Geometry check sheet. Reference: drawing and pictorial views, mm from the part's lowest x, y, z. A direction names the side the tool comes from. Give positions to 0.01 mm unless a question says otherwise; leave off trailing zeros. Write each loop counter-clockwise with the first axis right and the second up, starting at its lowest first coordinate (ties: lowest second). Pieces come first, ordered by that corner, then holes. Notation, with made-up numbers: M 43.5,-2.75 L 101.5,-2.75 A17 ccw 101.5,16.25 Z; hole C 52,-31.75 d7. An arc over 180 degrees is marked long. Write each question's results on one line, items separated by ' | '. Start each with the question number.
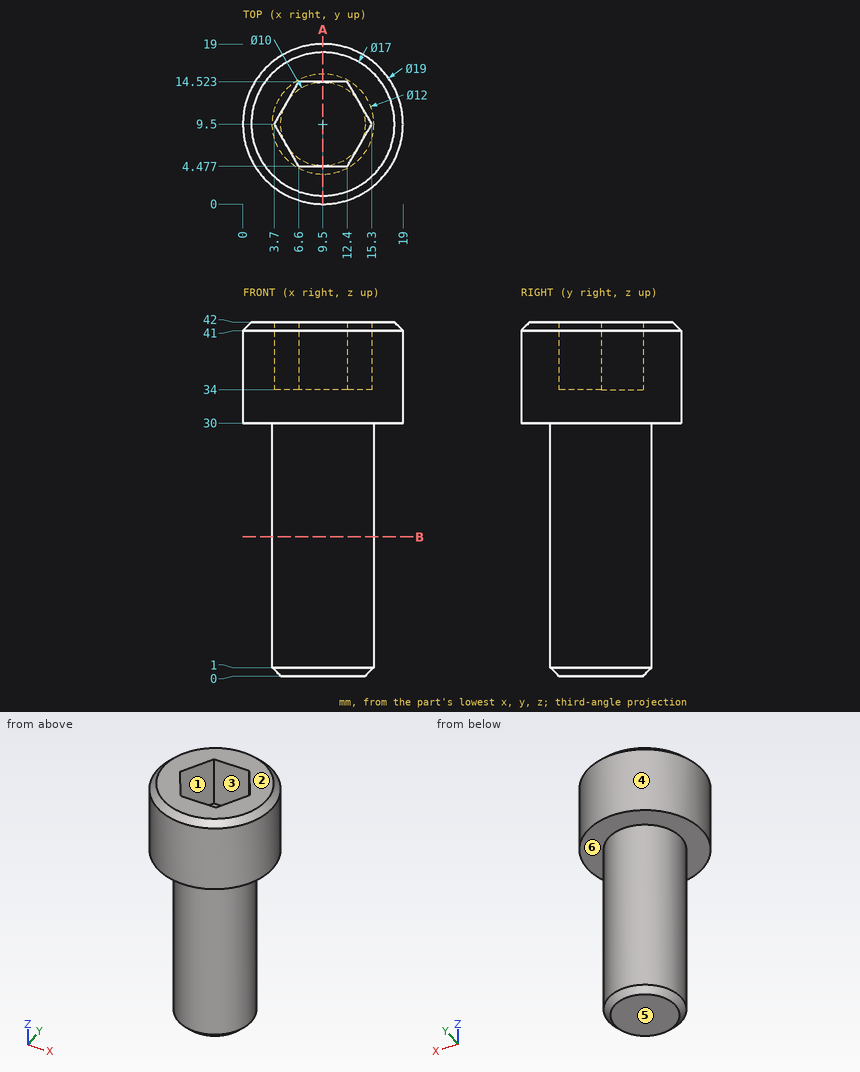
Q1. Section check B-B on z = 16.5. Record the boundary of the cut face in (x, y), plus the area to 3 significant figures.
Q2. Depth check by flat-ended pin: pin 1 Ø3 at (x, y) = (12, 9) entering from +Z; pin 2 Ø3 at (x, y) = (8, 17) entering from -Z; pin 3 Ø1.5 at (y, z) = (13, 35.5) entering from -X. Enter the tip coordinate at first touch or a pass-through.
Q3. Scan lines: L1, parallel to Z at x = 5.75, y = 4.5; L2, parallel to Y at x = 8, z = 21; L3, parallel to Y at x = 4.25, z = 36. Record each from-to range of solid material in increasing order.
Q4. Section check A-A on x = 9.5. Record the boundary of the cut face in (y, z).
Q5. Tool access check on the marked faces 5 and 6. Record the directions out of +Z, -Z, +X, -X, +Y, -Y that give a thin tool (end or side, any length) a straight path to the whole face; none if there is none.
Q6. Release check for a two-part mould opening along X. For the marked faces 1, 2, 3 and 4 record: pulls with the +X half, pulls with the -X half, needs draft (parallel to the pull), parting line crosses it, or undercut.
Check result:
1) outline: C 9.5,9.5 d12 | area: 113 mm^2
2) pin 1: z = 34 | pin 2: z = 30 | pin 3: x = 0.41
3) L1: 30 to 42 | L2: 3.69 to 15.31 | L3: 1.58 to 8.55, 10.45 to 17.42
4) outline: M 0,30 L 3.5,30 L 3.5,1 L 4.5,0 L 14.5,0 L 15.5,1 L 15.5,30 L 19,30 L 19,41 L 18,42 L 14.52,42 L 14.52,34 L 4.48,34 L 4.48,42 L 1,42 L 0,41 Z
5) face 5: -Z, +X, -X, +Y, -Y | face 6: -Z
6) face 1: undercut | face 2: needs draft | face 3: undercut | face 4: parting line crosses it
